Geometry check sheet. Reference: the model listing, model coordinates, mm. A direction names the side the tool comes from. Coordinates: 2 decimals unless noted, no trailing zeros. Loops run counter-clockwise (first coordinate to the right, second up) from the corner with the lowest first, then second, coordinate; pieces in that order, holes last. Notation, with made-up numbers: (59.5, -9) - (83.5, -9) arc R16 ccw to (83.5, 10) - close; hole circle Ø1 at (-21.5, -8). An arc over 180 degrees is marked (long way). One line per item, written item: value.
from build123d import *

# Parameters (mm, degrees)
EXTRUSION1_DEPTH                  = 2.9
ESQUISSE2_W                       = 10.2
ESQUISSE2_H                       = 1.4
EXTRUSION2_DEPTH                  = 2.7
CONG_1_R                          = 1
ESQUISSE3_W                       = 20.466591469
ESQUISSE3_H                       = 12.2
ESQUISSE3_W_2                     = 21.733408531
ESQUISSE3_W_3                     = 12.4
ESQUISSE3_H_2                     = 13.863540316
ENL_V_MAT_EXTRU_1_DEPTH           = 1
ESQUISSE4_R                       = 2.8
ENL_V_MAT_EXTRU_2_DEPTH           = 2
EXTRUSION3_DEPTH                  = 1
EXTRUSION3_DEPTH_BACK             = 1
ESQUISSE5_R                       = 4.6
CONG_2_R                          = 1
ESQUISSE6_R                       = 1.3
ENL_V_MAT_EXTRU_4_DEPTH           = 51.085976067
EXTRUSION4_DEPTH                  = 1
R_P_TITION_LIN_AIRE1_COUNT        = 2
R_P_TITION_LIN_AIRE1_PITCH        = 6
R_P_TITION_LIN_AIRE2_COUNT        = 2
R_P_TITION_LIN_AIRE2_PITCH        = 36.6
R_P_TITION_LIN_AIRE2_COPY_1_DEPTH = 1


with BuildPart() as part:
    # Esquisse1 → Extrusion1 (new body)
    with BuildSketch(Plane.XY):
        with BuildLine():
            Line((23.2, -23.001261172), (23.2, -15.001261172))
            Line((23.2, -15.001261172), (27, -15.001261172))
            ThreePointArc((27, -15.001261172), (34.071067812, -12.072328984), (37, -5.001261172))
            Line((37, -5.001261172), (37, 20.998738828))
            ThreePointArc((37, 20.998738828), (34.071067812, 28.069806639), (27, 30.998738828))
            Line((27, 30.998738828), (-27, 30.998738828))
            ThreePointArc((-27, 30.998738828), (-34.071067812, 28.069806639), (-37, 20.998738828))
            Line((-37, 20.998738828), (-37, -5.001261172))
            ThreePointArc((-37, -5.001261172), (-34.071067812, -12.072328984), (-27, -15.001261172))
            Line((-27, -15.001261172), (-23.2, -15.001261172))
            Line((-23.2, -15.001261172), (-23.2, -23.001261172))
            ThreePointArc((-23.2, -23.001261172), (-18.6, -27.601261172), (-14, -23.001261172))
            Line((-14, -23.001261172), (-14, -15.001261172))
            Line((-14, -15.001261172), (14, -15.001261172))
            Line((14, -15.001261172), (14, -23.001261172))
            ThreePointArc((14, -23.001261172), (18.6, -27.601261172), (23.2, -23.001261172))
        make_face()
    extrude(amount=-EXTRUSION1_DEPTH)

    # Esquisse2 → Extrusion2 (add)
    with BuildSketch(Plane(origin=(0, 30.998738828, 0), x_dir=(-1, 0, 0), z_dir=(0, 1, 0))):
        with Locations((-18.6, -2.2)):
            Rectangle(ESQUISSE2_W, ESQUISSE2_H)
        with Locations((18.6, -2.2)):
            Rectangle(ESQUISSE2_W, ESQUISSE2_H)
    extrude(amount=EXTRUSION2_DEPTH)

    # Congé1
    cong_1_edges = [part.edges().sort_by_distance(p)[0] for p in [
        (23.7, 33.698738828, -2.2),
        (13.5, 33.698738828, -2.2),
        (-23.7, 33.698738828, -2.2),
        (-13.5, 33.698738828, -2.2),
    ]]
    fillet(cong_1_edges, radius=CONG_1_R)

    # Esquisse3 → Enlèv. mat.-Extru.1 (cut)
    with BuildSketch(Plane(origin=(0, 0, -2.9), x_dir=(-1, 0, 0), z_dir=(0, 0, -1))):
        with BuildLine():
            Line((35.6, -5.001261172), (35.6, 0.735198512))
            Line((35.6, 0.735198512), (23.2, 0.735198512))
            Line((23.2, 0.735198512), (23.2, -13.601261172))
            Line((23.2, -13.601261172), (27, -13.601261172))
            ThreePointArc((27, -13.601261172), (33.081118318, -11.082379491), (35.6, -5.001261172))
        make_face()
        with BuildLine():
            Line((21.8, -23.001261172), (21.8, -13.601261172))
            Line((21.8, -13.601261172), (21.8, 0.735198512))
            Line((21.8, 0.735198512), (0.066591469, 0.735198512))
            Line((0.066591469, 0.735198512), (0.066591469, -11.464801488))
            Line((0.066591469, -11.464801488), (15.4, -11.464801488))
            Line((15.4, -11.464801488), (15.4, -23.001261172))
            ThreePointArc((15.4, -23.001261172), (18.6, -26.201261172), (21.8, -23.001261172))
        make_face()
        with BuildLine():
            Line((-15.4, -11.464801488), (-1.333408531, -11.464801488))
            Line((-1.333408531, -11.464801488), (-1.333408531, 0.735198512))
            Line((-1.333408531, 0.735198512), (-21.8, 0.735198512))
            Line((-21.8, 0.735198512), (-21.8, -13.601261172))
            Line((-21.8, -13.601261172), (-21.8, -23.001261172))
            ThreePointArc((-21.8, -23.001261172), (-18.6, -26.201261172), (-15.4, -23.001261172))
            Line((-15.4, -23.001261172), (-15.4, -11.464801488))
        make_face()
        with BuildLine():
            Line((-27, -13.601261172), (-23.2, -13.601261172))
            Line((-23.2, -13.601261172), (-23.2, 0.735198512))
            Line((-23.2, 0.735198512), (-35.6, 0.735198512))
            Line((-35.6, 0.735198512), (-35.6, -5.001261172))
            ThreePointArc((-35.6, -5.001261172), (-33.081118318, -11.082379491), (-27, -13.601261172))
        make_face()
        with BuildLine():
            Line((-35.6, 20.998738828), (-35.6, 17.398738828))
            Line((-35.6, 17.398738828), (-23.2, 17.398738828))
            Line((-23.2, 17.398738828), (-23.2, 29.598738828))
            Line((-23.2, 29.598738828), (-27, 29.598738828))
            ThreePointArc((-27, 29.598738828), (-33.081118318, 27.079857146), (-35.6, 20.998738828))
        make_face()
        with BuildLine():
            Line((27, 29.598738828), (23.2, 29.598738828))
            Line((23.2, 29.598738828), (23.2, 17.398738828))
            Line((23.2, 17.398738828), (35.6, 17.398738828))
            Line((35.6, 17.398738828), (35.6, 20.998738828))
            ThreePointArc((35.6, 20.998738828), (33.081118318, 27.079857146), (27, 29.598738828))
        make_face()
        with Locations((-11.566704266, 23.498738828)):
            Rectangle(ESQUISSE3_W, ESQUISSE3_H)
        with Locations((10.933295734, 23.498738828)):
            Rectangle(ESQUISSE3_W_2, ESQUISSE3_H)
        with Locations((-29.4, 9.06696867)):
            Rectangle(ESQUISSE3_W_3, ESQUISSE3_H_2)
        with Locations((-11.566704266, 9.06696867)):
            Rectangle(ESQUISSE3_W, ESQUISSE3_H_2)
        with Locations((10.933295734, 9.06696867)):
            Rectangle(ESQUISSE3_W_2, ESQUISSE3_H_2)
        with Locations((29.4, 9.06696867)):
            Rectangle(ESQUISSE3_W_3, ESQUISSE3_H_2)
    extrude(amount=-ENL_V_MAT_EXTRU_1_DEPTH, mode=Mode.SUBTRACT)

    # Esquisse4 → Enlèv. mat.-Extru.2 (cut)
    with BuildSketch(Plane.XY):
        with Locations((-18.6, -19.001261172)):
            Circle(ESQUISSE4_R)
        with Locations((18.6, -19.001261172)):
            Circle(ESQUISSE4_R)
    extrude(amount=-ENL_V_MAT_EXTRU_2_DEPTH, mode=Mode.SUBTRACT)

    # Esquisse5 → Extrusion3 (add, two sides: drawn at the far end of the back side and taken through both)
    with BuildSketch(Plane(origin=(0, 0, -2.9), x_dir=(-1, 0, 0), z_dir=(0, 0, -1)).offset(-EXTRUSION3_DEPTH_BACK)):
        with Locations((-18.6, -19.001261172)):
            Circle(ESQUISSE5_R)
        with Locations((18.6, -19.001261172)):
            Circle(ESQUISSE5_R)
    extrude(amount=EXTRUSION3_DEPTH + EXTRUSION3_DEPTH_BACK)

    # Congé2
    cong_2_edges = [part.edges().sort_by_distance(p)[0] for p in [
        (23.2, -19.001261172, -3.9),
        (-14, -19.001261172, -3.9),
    ]]
    fillet(cong_2_edges, radius=CONG_2_R - 0.0001)  # a hair under: the kernel refuses the full size

    # Esquisse6 → Enlèv. mat.-Extru.4 (cut, through all)
    with BuildSketch(Plane.XY.offset(-1.9)):
        with Locations((18.6, -19.001261172)):
            Circle(ESQUISSE6_R)
        with Locations((-18.6, -19.001261172)):
            Circle(ESQUISSE6_R)
    extrude(amount=-ENL_V_MAT_EXTRU_4_DEPTH, mode=Mode.SUBTRACT)

    # Esquisse7 → Extrusion4 (add)
    with BuildSketch(Plane.ZY.offset(-21.8)):
        Polygon((-2.9, 32.698738828), (-3.9, 32.334768593), (-3.9, 29.534768593), (-1.9, 27.398738828), (-1.9, 29.598738828), (-2.9, 29.598738828), align=None)
    extrusion4 = extrude(amount=EXTRUSION4_DEPTH)

    # Répétition linéaire1: Extrusion4 ×2
    with Locations(*[(-i * R_P_TITION_LIN_AIRE1_PITCH, 0, 0) for i in range(1, R_P_TITION_LIN_AIRE1_COUNT)]):
        add(extrusion4)

    # Répétition linéaire2: Extrusion4 ×2
    with Locations(*[(-i * R_P_TITION_LIN_AIRE2_PITCH, 0, 0) for i in range(1, R_P_TITION_LIN_AIRE2_COUNT)]):
        add(extrusion4)

    # Répétition linéaire2 copy 1 sketch → Répétition linéaire2 copy 1 (add)
    with BuildSketch(Plane.ZY.offset(20.8)):
        Polygon((-2.9, 32.698738828), (-3.9, 32.334768593), (-3.9, 29.534768593), (-1.9, 27.398738828), (-1.9, 29.598738828), (-2.9, 29.598738828), align=None)
    extrude(amount=R_P_TITION_LIN_AIRE2_COPY_1_DEPTH)


solid = part.part
(1) Go/stop test with flat-tipped pins: pin 1 Ø1 at (y, z) = (-19.5, -3) entering from -X; pin 2 Ø0.8 at (y, z) = (25, -2.5) entering from -X; pin 3 Ø0.7 at (y, z) = (32, -2.5) entering from +X. Record where each tip stops, or that it passes through.
Reply:
pin 1: x = -23.2
pin 2: x = -36.33
pin 3: x = 23.7
(2) Release check for a two-part mould opening along Y. For faces 5 (the face through (15.31, 28.48, -2.91)), 6 (the face through (18.5, -27.6, -1.4)), 7 (the face through (-14, -19, -1)) record: pulls with the +Y half, pulls with the -Y half, needs draft (parallel to the pull), parting line crosses it, or undercut.
Reply:
face 5: undercut
face 6: pulls with the -Y half
face 7: needs draft
(3) Access from +Z, -Z, +X, -X, +Y, -Y to the whole of each face (thin tool, end or side, straight path). Record for faces 1 (the face through (18.2, -26.5, -2.9)), 2 (the face through (-23.2, -19, -1)), 3 (the face through (-21.29, 28.48, -2.91)), 4 (the face through (17, -20, -1.9)).
Reply:
face 1: -Z, -Y
face 2: +Z, -Z, -X, -Y
face 3: -Z
face 4: +Z
(4) Material ranges on probe 1 along X at (y, z) = (-4, -2.4); probe 2 along Y at (x, z) = (1.5, -2.05); probe 3 along Y at (x, z) = (-18.6, -2.45), recorded low to high. Write a range as from..to.
Reply:
probe 1: -37..-35.6, -23.2..-21.8, -0.07..1.33, 21.8..23.2, 35.6..37
probe 2: -15..-11.46, 0.74..2.14, 16..17.4, 29.6..31
probe 3: -27.6..-26.2, -23.6..-20.3, -17.7..-14.4, 0.74..2.14, 16..17.4, 29.6..33.7
(5) Cross-section at B-B on y = 11. Record the cut outline in (x, z), and give its area (3 significant figures).
Reply:
outline: (-37, -2.9) - (-35.6, -2.9) - (-35.6, -1.9) - (-23.2, -1.9) - (-23.2, -2.9) - (-21.8, -2.9) - (-21.8, -1.9) - (-0.07, -1.9) - (-0.07, -2.9) - (1.33, -2.9) - (1.33, -1.9) - (21.8, -1.9) - (21.8, -2.9) - (23.2, -2.9) - (23.2, -1.9) - (35.6, -1.9) - (35.6, -2.9) - (37, -2.9) - (37, 0) - (-37, 0) - close
area: 148 mm2
